Could you check a few things on this model? Use its own coordinates, in mm. A direction names the side the tool comes from. Round coordinates to 2 decimals unless told otherwise and drop trailing zeros. Write each loop counter-clockwise with the first axis right and the second up, starting at its lowest first coordinate (ties: lowest second). Pieces come first, ordered by that corner, then holes. Notation, with made-up numbers: (-24.5, 36.25) -> (-8.5, 36.25) arc R18 ccw to (-8.5, 61.25) -> close; hole circle Ø5 at (-35.75, -36.75). An arc over 180 degrees is marked (long way). Return JSON: item names as keys, results as strings.
Autodesk Inventor part; units mm, degrees
ref_plane "YZ Plane" through (0, 0, 0) normal (1, 0, 0) x (0, 1, 0)
ref_plane "XZ Plane" through (0, 0, 0) normal (0, 1, 0) x (-1, 0, 0)
ref_plane "XY Plane" through (0, 0, 0) normal (0, 0, 1) x (1, 0, 0)
sketch "Sketch1" plane through (0, 0, 0) normal (0, 0, 1) x (1, 0, 0)
  line L0 (0, 0) -> (1.6, 0)
  line L1 (1.6, 0) -> (1.6, 23.05)
  line L2 (1.6, 23.05) -> (0, 23.05)
  line L3 (0, 23.05) -> (0, 0)
  line L4 (0, 0) -> (19.97, 0)
  line L5 (19.97, 0) -> (19.97, 1.6)
  line L6 (19.97, 1.6) -> (0, 1.6)
  line L7 (0, 1.6) -> (0, 0)
  line L8 (0, 23.05) -> (19.97, 23.05)
  line L9 (19.97, 23.05) -> (19.97, 21.45)
  line L10 (19.97, 21.45) -> (0, 21.45)
  line L11 (0, 21.45) -> (0, 23.05)
  line L12 (19.97, 0) -> (18.37, 0)
  line L13 (18.37, 0) -> (18.37, 23.05)
  line L14 (18.37, 23.05) -> (19.97, 23.05)
  line L15 (19.97, 23.05) -> (19.97, 0)
  dimension "d0" = 1.6
  dimension "d1" = 1.6
  dimension "d2" = 1.6
  dimension "d3" = 1.6
  dimension "d4" = 19.85
  dimension "d5" = 16.77
extrude "Extrusion1" add sketch "Sketch1" along normal blind 35.48 contours L3 L6 L1 L0 | L1 L6 L13 L4 | L3 L10 L1 L6 | L13 L6 L5 L4 | L3 L2 L1 L10 | L1 L8 L13 L10 | L13 L10 L15 L6 | L13 L8 L9 L10
sketch "Sketch2" plane through (0, 0, 35.48) normal (0, 0, 1) x (1, 0, 0)
  line L0 (18.37, 21.45) -> (18.37, 1.6)
  line L1 (18.37, 1.6) -> (1.6, 1.6)
  line L2 (1.6, 1.6) -> (1.6, 21.45)
  line L3 (1.6, 21.45) -> (18.37, 21.45)
  line L4 (19.97, 23.05) -> (0, 23.05)
  line L5 (0, 23.05) -> (0, 0)
  line L6 (0, 0) -> (19.97, 0)
  line L7 (19.97, 0) -> (19.97, 23.05)
  line L8 (19.97, 0) -> (19.97, 23.05)
  line L9 (0, 0) -> (19.97, 0)
  line L10 (19.97, 0) -> (19.97, 1.6)
  line L11 (19.97, 1.6) -> (0, 1.6)
  line L12 (0, 1.6) -> (0, 0)
  line L13 (18.37, 1.6) -> (18.37, 0)
  line L14 (0, 0) -> (19.97, 0)
  line L15 (1.6, 1.6) -> (1.6, 0)
  line L16 (1.6, 1.6) -> (18.37, 1.6)
  line L17 (18.37, 1.6) -> (18.37, 0)
  line L18 (18.37, 0) -> (1.6, 0)
  line L19 (1.6, 0) -> (1.6, 1.6)
ref_plane "Work Plane1" through (0, 0, 16) normal (0, 0, -1) x (-1, 0, 0)
sketch "Sketch3" plane through (0, 0, 0) normal (-1, 0, 0) x (0, 0, 1)
  line L0 (0, 0) -> (35.48, 0)
  line L1 (1.7, 0) -> (2.5, 0.8)
  line L2 (1.7, 0) -> (2.8314, 0) construction
  line L3 (2.5, 0.8) -> (4.1, 0.8)
  line L4 (4.1, 0.8) -> (4.9, 0)
  line L5 (0, 23.05) -> (0, 0)
  point P0 (16, 0)
  dimension "d11" = 45
  dimension "d12" = 1.6
  dimension "d13" = 0.8
  dimension "d14" = 45
  dimension "d15" = 2.5
extrude "Extrusion3" cut sketch "Sketch3" against normal up to next
extrude "Extrusion4" cut sketch "Sketch2" against normal up to surface (19.48 mm away) contours L13 L6 L15 L1
ref_plane "Midway" through (0, 0, 17.74) normal (0, 0, -1) x (-1, 0, 0)
mirror "Mirror1" about plane through (0, 0, 17.74) normal (0, 0, -1) of "Extrusion3"
properties part number "CarEngineHousing"
1) I want a section at A-A, the plane z = 6.5. Please give me the cut outline in (x, y), and give its area (3 significant figures).
Return value:
{"outline": "(0, 0) -> (19.97, 0) -> (19.97, 23.05) -> (0, 23.05) -> close; hole (1.6, 1.6) -> (18.37, 1.6) -> (18.37, 21.45) -> (1.6, 21.45) -> close", "area": "127 mm²"}
2) Thinking about a two-plate mould opening in X: for faces 4 (the face through (1, 0.8, 32)), 5 (the face through (10, 21.45, 17)), 6 (the face through (0, 12, 17)), which applies, pulls with the +X half, pulls with the -X half, needs draft (parallel to the pull), parting line crosses it, or undercut?
Return value:
{"face 4": "needs draft", "face 5": "undercut", "face 6": "pulls with the -X half"}
3) I want a section at C-C, the plane y = 10.75. Please give me the cut outline in (x, z), and give its area (3 significant figures).
Return value:
{"outline": "(0, 0) -> (1.6, 0) -> (1.6, 35.48) -> (0, 35.48) -> close; (18.37, 0) -> (19.97, 0) -> (19.97, 35.48) -> (18.37, 35.48) -> close", "area": "114 mm²"}
4) I want a section at D-D, the plane z = 17. Please give me the cut outline in (x, y).
Return value:
{"outline": "(0, 0) -> (1.6, 0) -> (1.6, 21.45) -> (18.37, 21.45) -> (18.37, 0) -> (19.97, 0) -> (19.97, 23.05) -> (0, 23.05) -> close"}
5) If I drill on probe 1 along Y at (x, z) = (17, 6.5); probe 2 along X at (y, z) = (17.25, 23.5); probe 3 along Y at (x, z) = (15, 3), over which ranges is the centre line in solid material (lowest first)? Write a range as [from, to].
Return value:
{"probe 1": "[0, 1.6], [21.45, 23.05]", "probe 2": "[0, 1.6], [18.37, 19.97]", "probe 3": "[0.8, 1.6], [21.45, 23.05]"}
6) I want a section at B-B, the plane x = 14.5. Please give me the cut outline in (y, z).
Return value:
{"outline": "(0, 0) -> (1.6, 0) -> (1.6, 16) -> (0, 16) -> (0, 4.9) -> (0.8, 4.1) -> (0.8, 2.5) -> (0, 1.7) -> close; (21.45, 0) -> (23.05, 0) -> (23.05, 35.48) -> (21.45, 35.48) -> close"}
7) Will these pins go through, and if not, where does the flat tip stop? pin 1 Ø8 at (x, y) = (6.5, 20.5) entering from +Z; pin 2 Ø1.3 at (x, z) = (12.5, 3.5) entering from -Y; pin 3 Ø1.8 at (x, y) = (6.5, 1) entering from +Z.
Return value:
{"pin 1": "z = 35.48", "pin 2": "y = 0.75", "pin 3": "z = 16"}
8) For faces 1 (the face through (10, 1.6, 8)), 2 (the face through (10, 1, 16)), 3 (the face through (9.8, 0.4, 4.5)), which set-ups out of +Z, -Z, +X, -X, +Y, -Y let a thin tool reach every point of the face, with its end or its side?
Return value:
{"face 1": "+Z, -Z", "face 2": "+Z, -Y", "face 3": "+X, -X, -Y"}
